The drawing under review shows one solid part. Ordinate dimensions are in mm from its lowest x, y, z. Give positions to 0.01 mm unless a question says otherwise; leave off trailing zeros. Write each loop counter-clockwise with the first axis right and the second up, starting at its lowest first coordinate (ties: lowest second). Pieces come first, ordered by that corner, then holes. Notation, with made-up numbers: (83, 7) -> (101, 7) arc R7 ccw to (101, 13) -> close; hole circle Ø10 at (-18.75, -11.75). An arc over 180 degrees is marked (long way). Use CSV: the item, a comma, the result in double quotes.
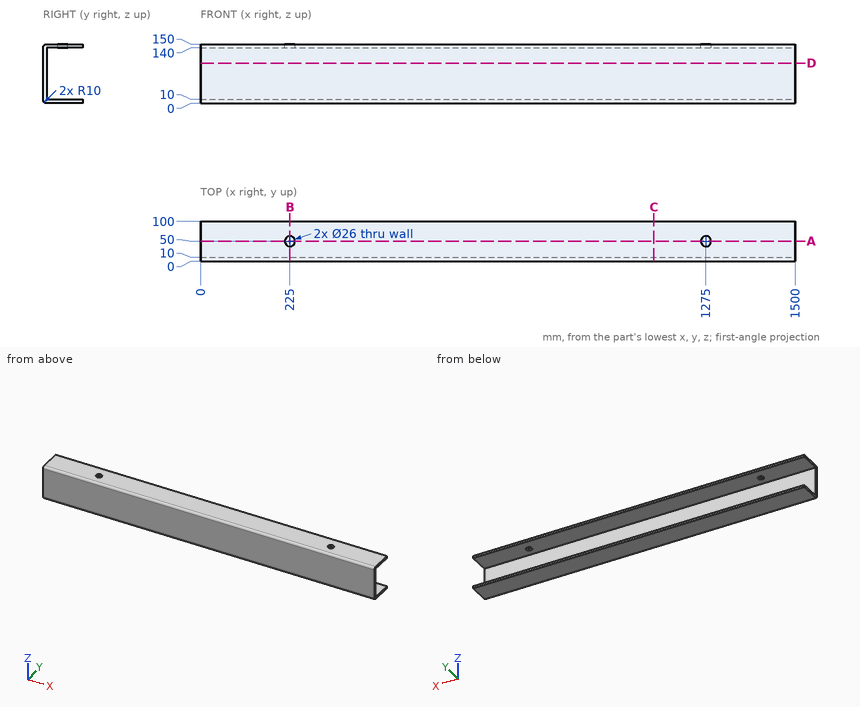
(1) Take a section at A-A (y = 50). Write out the cut boundary in (x, z).
Established:
outline,"(0, 0) -> (1500, 0) -> (1500, 10) -> (0, 10) -> close; (0, 140) -> (212, 140) -> (212, 150) -> (0, 150) -> close; (238, 140) -> (1262, 140) -> (1262, 150) -> (238, 150) -> close; (1288, 140) -> (1500, 140) -> (1500, 150) -> (1288, 150) -> close"
(2) Take a section at C-C (x = 1144). Write out the cut boundary in (y, z).
Established:
outline,"(0, 10) arc R10 ccw to (10, 0) -> (100, 0) -> (100, 10) -> (10, 10) -> (10, 140) -> (100, 140) -> (100, 150) -> (10, 150) arc R10 ccw to (0, 140) -> close"
(3) For line 1 along Z through (x, y) = (597.5, 38); line 2 along Y through (x, z) = (535, 40); line 3 along Y through (x, z) = (1275, 143.5), list the stretches that pass through material, from the lowest coordinate up. Write a range as [from, to].
Established:
line 1,"z = [0, 10], [140, 150]"
line 2,"y = [0, 10]"
line 3,"y = [0.63, 37], [63, 100]"
(4) Clearance check with a flat-ended pin moving along its axis: pin 1 (12 mm diameter, centred on x = 1043.5, z = 50.5, fed in from +Y). State where the tip first meets the part, or that it passes through.
Established:
pin 1,"stops at y = 10"
(5) Take a section at D-D (z = 102). Write out the cut boundary in (x, y), then the cut area to 3 significant figures.
Established:
outline,"(0, 0) -> (1500, 0) -> (1500, 10) -> (0, 10) -> close"
area,"15,000 mm2"
(6) Take a section at B-B (x = 225). Write out the cut boundary in (y, z).
Established:
outline,"(0, 10) arc R10 ccw to (10, 0) -> (100, 0) -> (100, 10) -> (10, 10) -> (10, 140) -> (37, 140) -> (37, 150) -> (10, 150) arc R10 ccw to (0, 140) -> close; (63, 140) -> (100, 140) -> (100, 150) -> (63, 150) -> close"
